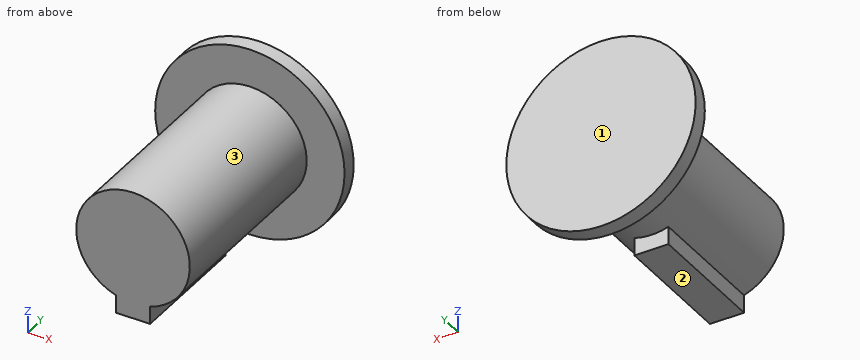
from build123d import *

# Parameters (mm, degrees)
SKETCH_1_R      = 3
EXTRUDE_2_DEPTH = 11
EXTRUDE_3_DEPTH = 6.6
SKETCH_3_R      = 5
EXTRUDE_4_DEPTH = 0.8


with BuildPart() as part:
    # Sketch 1 → Extrude 2 (new body)
    with BuildSketch(Plane(origin=(0, 0, 0), x_dir=(1, 0, 0), z_dir=(0, 1, 0))):
        with Locations(Location((0, 0, 0), (0, 0, 270))):
            Circle(SKETCH_1_R)
    extrude(amount=EXTRUDE_2_DEPTH)

    # Sketch 1_3 → Extrude 3 (add)
    with BuildSketch(Plane(origin=(0, 0, 0), x_dir=(1, 0, 0), z_dir=(0, 1, 0))):
        with BuildLine():
            Line((-0.9, 3.8), (-0.9, 2.861817604))
            ThreePointArc((-0.9, 2.861817604), (0, 3), (0.9, 2.861817604))
            Line((0.9, 2.861817604), (0.9, 3.8))
            Line((0.9, 3.8), (-0.9, 3.8))
        make_face()
    extrude(amount=EXTRUDE_3_DEPTH)

    # Sketch 3 → Extrude 4 (add)
    with BuildSketch(Plane(origin=(0, 11, 0), x_dir=(1, 0, 0), z_dir=(0, 1, 0))):
        with Locations(Location((0, 0, 0), (0, 0, 270))):
            Circle(SKETCH_3_R)
    extrude(amount=-EXTRUDE_4_DEPTH)


solid = part.part
Geometry: final body of the model. Coordinates: model frame, mm. Face numbers are marked on the shaded views. Round coordinates to 2 decimals unless told otherwise and drop trailing zeros. Order: outer loops, then holes, each group sorted by start corner. A loop starts at its lowest first (then second) coordinate and runs counter-clockwise, first axis right, second up.
Q1. Section C-C, the plane y = 7. Output: boundary loops of the cut face in (x, z).
Result sheet:
outline: circle Ø6 at (0, 0)
Q2. Mould query, pull axis Z, two halves, no side actions, for the marked faces 1, 2 and 3. Classes: released by +Z, released by -Z, zero draft, split by the parting line, or undercut.
Result sheet:
face 1: zero draft
face 2: released by -Z
face 3: split by the parting line
Q3. Pin query (flat end, axial travel): pin 1 (4 mm diameter, centred on y = 7, z = 2, fed in from -X); pin 2 (2 mm diameter, centred on x = 1, y = 4, fed in from +Z); pin 3 (1 mm diameter, centred on y = 4.5, z = -3, fed in from +X). Return the tip coordinate at first contact, or that it passes through.
Result sheet:
pin 1: stops at x = -3
pin 2: stops at z = 3
pin 3: stops at x = 1.66
Q4. Section A-A, the plane x = 0. Output: boundary loops of the cut face in (y, z).
Result sheet:
outline: (0, -3.8) - (6.6, -3.8) - (6.6, -3) - (10.2, -3) - (10.2, -5) - (11, -5) - (11, 5) - (10.2, 5) - (10.2, 3) - (0, 3) - close
Q5. Material intervals for probe 1 along Y at (x, z) = (4.25, -2); probe 2 along Z at (x, y) = (-2, 10); probe 3 along X at (y, z) = (7, 1.5), sorted ascending.
Result sheet:
probe 1: y = 10.2 to 11
probe 2: z = -2.24 to 2.24
probe 3: x = -2.6 to 2.6
Q6. Section B-B, the plane z = 0. Output: boundary loops of the cut face in (x, y), and give its area (3 significant figures).
Result sheet:
outline: (-5, 10.2) - (-3, 10.2) - (-3, 0) - (3, 0) - (3, 10.2) - (5, 10.2) - (5, 11) - (-5, 11) - close
area: 69.2 mm2
Q7. Section D-D, the plane z = -2. Output: boundary loops of the cut face in (x, y), and give its area (3 significant figures).
Result sheet:
outline: (-4.58, 10.2) - (-2.24, 10.2) - (-2.24, 0) - (2.24, 0) - (2.24, 10.2) - (4.58, 10.2) - (4.58, 11) - (-4.58, 11) - close
area: 52.9 mm2
